```python
from build123d import *

# Parameters (mm, degrees)
SKETCH1_W            = 2280
SKETCH1_H            = 135
BASE_FLANGE1_DEPTH   = 12
EDGE_FLANGE1_START   = -1140
EDGE_FLANGE1_DEPTH   = 2280
EDGE_FLANGE1_2_DEPTH = 2280


# Read off the part's stored shape, not the designer's step: Edge-Flange1
# Sheet-metal steps are written as plain solids
with BuildPart() as part:
    # Sketch1 → Base-Flange1 (new body)
    with BuildSketch(Plane(origin=(0, 0, 0), x_dir=(1, 0, 0), z_dir=(0, 1, 0))):
        Rectangle(SKETCH1_W, SKETCH1_H)
    extrude(amount=-BASE_FLANGE1_DEPTH)

    # Edge-Flange1 outline → Edge-Flange1 (cut)
    with BuildSketch(Plane.YZ.offset(EDGE_FLANGE1_START)):
        with BuildLine():
            Line((0, -67.5), (-8.382685902, -52.980762114))
            ThreePointArc((-8.382685902, -52.980762114), (-11.07999731, -46.468876332), (-12, -39.480762114))
            Line((-12, -39.480762114), (-12, -67.5))
            Line((-12, -67.5), (0, -67.5))
        make_face()
    extrude(amount=EDGE_FLANGE1_DEPTH, mode=Mode.SUBTRACT)

    # Edge-Flange1 2 outline → Edge-Flange1 2 (add)
    with BuildSketch(Plane.YZ.offset(EDGE_FLANGE1_START)):
        with BuildLine():
            Line((0, -39.480762114), (0, -67.5))
            Line((0, -67.5), (3, -72.696152423))
            Line((3, -72.696152423), (13.392304845, -66.696152423))
            Line((13.392304845, -66.696152423), (2.009618943, -46.980762114))
            ThreePointArc((2.009618943, -46.980762114), (0.511112606, -43.36304779), (0, -39.480762114))
        make_face()
    extrude(amount=EDGE_FLANGE1_2_DEPTH)


solid = part.part
```
Build history of the part. All positions in model axes, mm. A direction names the side the tool comes from. Give positions to 0.01 mm unless a question says otherwise; leave off trailing zeros. Loops run counter-clockwise (first coordinate to the right, second up) from the corner with the lowest first, then second, coordinate; pieces in that order, holes last.
Item 1: Flat gauge pins, fed straight in: pin 1 (5 mm diameter, centred on x = 888.5, y = 7, fed in from +Z); pin 2 (6 mm diameter, centred on x = 618, y = 6, fed in from +Z); pin 3 (1.5 mm diameter, centred on x = 794.5, y = 3.5, fed in from +Z). Where does each tip first touch, or does it go through?
Answers follow:
pin 1: stops at z = -51.29
pin 2: stops at z = -48.7
pin 3: stops at z = -48.26
Item 2: Drill centre lines: line 1 (Y direction, x = -211.5, z = -21.5); line 2 (Z direction, x = -258, y = -8.5); line 3 (Y direction, x = 482, z = -46). Where is each one in solid material? Low to high.
Answers follow:
line 1: y = -12 to 0
line 2: z = -52.78 to 67.5
line 3: y = -11.2 to 1.49
Item 3: Slice it at A-A, the plane x = -553.5. List the corners of the cut face in (y, z), and give its area (3 significant figures).
Answers follow:
outline: (-12, -39.48) arc R27 ccw to (-8.38, -52.98) - (3, -72.7) - (13.39, -66.7) - (2.01, -46.98) arc R15 cw to (0, -39.48) - (0, 67.5) - (-12, 67.5) - close
area: 1,690 mm2
Item 4: Slice it at B-B, the plane z = 8. List the corners of the cut face in (x, y), and give its area (3 significant figures).
Answers follow:
outline: (-1140, -12) - (1140, -12) - (1140, 0) - (-1140, 0) - close
area: 27,400 mm2
Item 5: Which spindle directions (+Z, -Z, +X, -X, +Y, -Y) get a long thin tool onto all of the face, cutting with end or side? Do faces 1 (the face through (-16, 0, 13)), 2 (the face through (-16, -12, 13)). Say none if no direction does.
Answers follow:
face 1: +Z, +X, -X, +Y
face 2: +Z, -Z, +X, -X, -Y
Item 6: Slice it at C-C, the plane y = 7. List the corners of the cut face in (x, z).
Answers follow:
outline: (-1140, -70.39) - (1140, -70.39) - (1140, -55.62) - (-1140, -55.62) - close
